Part print with two shaded views. Sizes in mm from the minimum x, y, z corner. Give positions to 0.01 mm unless a question says otherwise; leave off trailing zeros. Loops run counter-clockwise (first coordinate to the right, second up) from the corner with the lowest first, then second, coordinate; pieces in that order, holes last. Notation, with made-up numbers: M -18.75,71 L 20.25,71 A19 ccw 20.25,84 Z; hole C -19,-9 d11. An arc over 180 degrees is marked long. Answer in a Markdown table with one row per item.
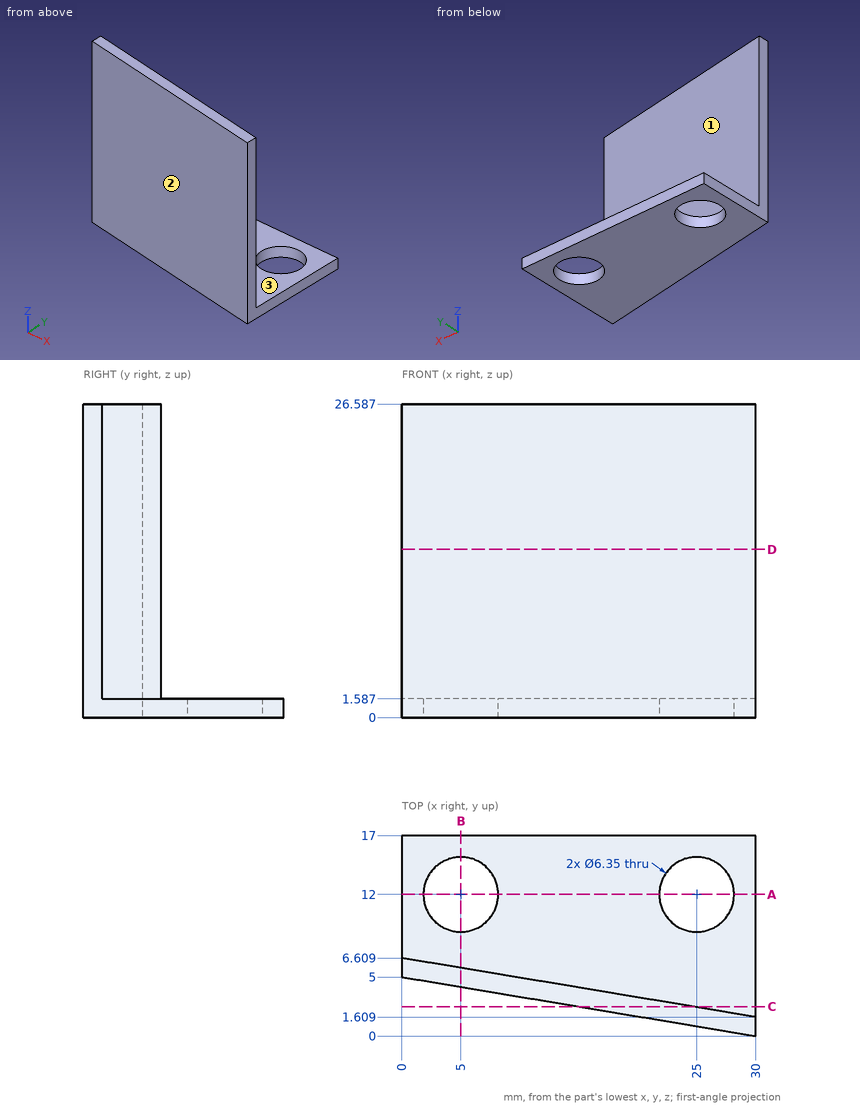
Q1. Saw through at B-B (x = 5). Give the cut face in (y, z) (1 decimal).
Reported:
| item | result |
|---|---|
| outline | M 4.2,0 L 8.8,0 L 8.8,1.6 L 5.8,1.6 L 5.8,26.6 L 4.2,26.6 Z; M 15.2,0 L 17,0 L 17,1.6 L 15.2,1.6 Z |
Q2. Saw through at A-A (y = 12). Give the cut face in (x, z) (1 decimal).
Reported:
| item | result |
|---|---|
| outline | M 0,0 L 1.8,0 L 1.8,1.6 L 0,1.6 Z; M 8.2,0 L 21.8,0 L 21.8,1.6 L 8.2,1.6 Z; M 28.2,0 L 30,0 L 30,1.6 L 28.2,1.6 Z |
Q3. Mould opens along X. For the marked faces 1, 2 and 3 say: released by +X, released by -X, zero draft, split by the parting line, or undercut.
Reported:
| item | result |
|---|---|
| face 1 | released by +X |
| face 2 | released by -X |
| face 3 | zero draft |
Q4. Drop flat-ended pins along their axis: pin 1 (5.5 mm diameter, centred on x = 25, y = 12, fed in from +Z); pin 2 (8 mm diameter, centred on x = 21.5, y = 8, fed in from +Z); pin 3 (12 mm diameter, centred on x = 7, z = 8, fed in from -Y); pin 4 (12 mm diameter, centred on x = 18.5, z = 19, fed in from -Y). Give the stop position or say it passes through.
Reported:
| item | result |
|---|---|
| pin 1 | through |
| pin 2 | z = 1.59 |
| pin 3 | y = 2.83 |
| pin 4 | y = 0.92 |
Q5. Probe probe 1 along Y at (x, z) = (5, 0.6) (1 decimal); probe 2 along Y at (x, z) = (25, 0.55) (1 decimal); probe 3 along Z at (x, y) = (1.5, 8.5). List the from-to ranges inside material, lowest first.
Reported:
| item | result |
|---|---|
| probe 1 | 4.2 to 8.8, 15.2 to 17 |
| probe 2 | 0.8 to 8.8, 15.2 to 17 |
| probe 3 | 0 to 1.59 |
Q6. Saw through at C-C (y = 2.5). Give the cut face in (x, z).
Reported:
| item | result |
|---|---|
| outline | M 15,0 L 30,0 L 30,1.59 L 24.66,1.59 L 24.66,26.59 L 15,26.59 Z |
Q7. Saw through at D-D (z = 14.25). Give the cut face in (x, y).
Reported:
| item | result |
|---|---|
| outline | M 0,5 L 30,0 L 30,1.61 L 0,6.61 Z |
